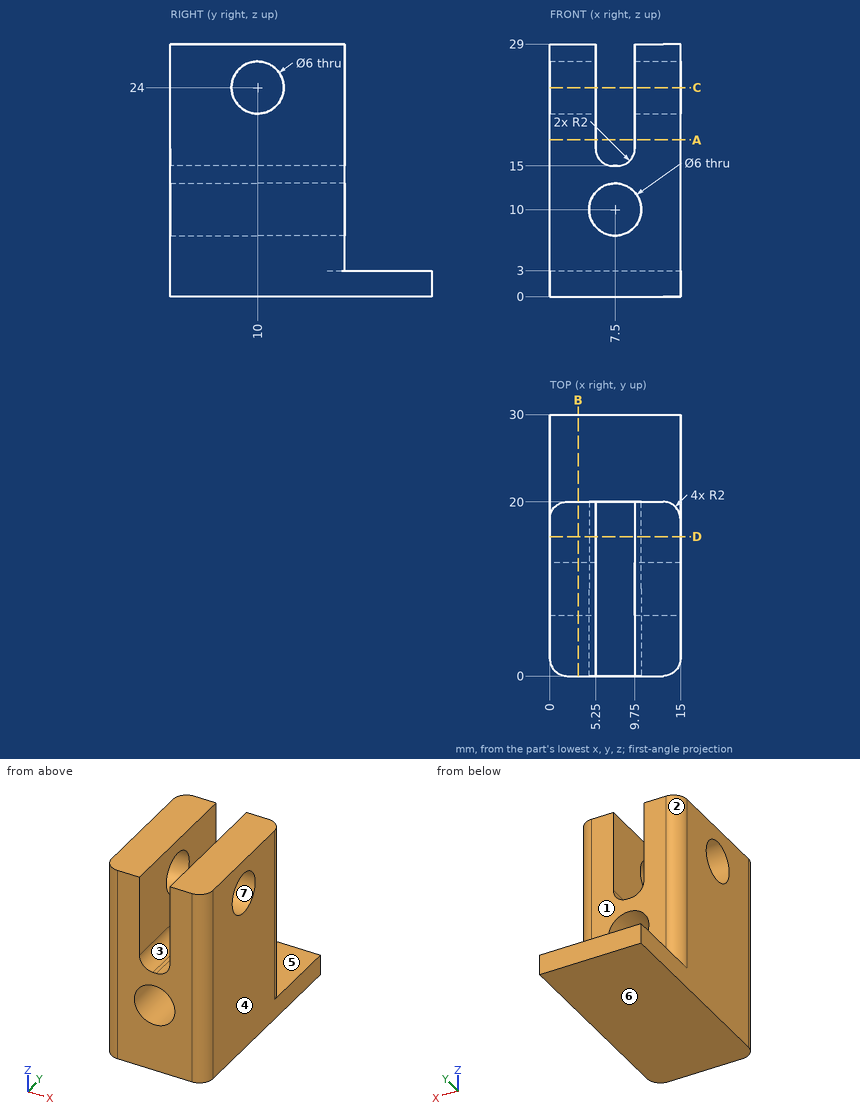
Print and shaded views of the part. All mm, measured from the part's lowest x, y and z. A direction names the side the tool comes from. Round coordinates to 2 decimals unless told otherwise and drop trailing zeros. Order: outer loops, then holes, each group sorted by start corner. A loop starts at its lowest first (then second) coordinate and runs counter-clockwise, first axis right, second up. Notation, with made-up numbers: (-38, 38.25) - (-14, 38.25) arc R35 ccw to (-14, 71.25) - close; hole circle Ø2 at (35.5, -25.75). An arc over 180 degrees is marked (long way). Use a Markdown table: item, result.
1) Saw through at C-C on z = 24. Write the cut outline in (x, y).
Recorded:
| item | result |
|---|---|
| outline | (0, 2) arc R2 ccw to (2, 0) - (5.25, 0) - (5.25, 7) - (0, 7) - close; (0, 13) - (5.25, 13) - (5.25, 20) - (2, 20) arc R2 ccw to (0, 18) - close; (9.75, 0) - (13, 0) arc R2 ccw to (15, 2) - (15, 7) - (9.75, 7) - close; (9.75, 13) - (15, 13) - (15, 18) arc R2 ccw to (13, 20) - (9.75, 20) - close |
2) Saw through at D-D on y = 16. Write the cut outline in (x, z), and give its area (3 significant figures).
Recorded:
| item | result |
|---|---|
| outline | (0, 0) - (15, 0) - (15, 29) - (9.75, 29) - (9.75, 17) arc R2 cw to (7.75, 15) - (7.25, 15) arc R2 cw to (5.25, 17) - (5.25, 29) - (0, 29) - close; hole circle Ø6 at (7.5, 10) |
| area | 345 mm² |
3) Tool access for the marked faces 1, 2 and 3: list every direction of +Z, -Z, +X, -X, +Y, -Y with a clear straight run to the whole face (end or side of a thin tool).
Recorded:
| item | result |
|---|---|
| face 1 | +Z, +X, -X, +Y |
| face 2 | +Z, -X, +Y |
| face 3 | +Z, +Y, -Y |
4) Saw through at B-B on x = 3.25. Write the cut outline in (y, z).
Recorded:
| item | result |
|---|---|
| outline | (0, 0) - (30, 0) - (30, 3) - (20, 3) - (20, 29) - (0, 29) - close; hole circle Ø6 at (10, 24) |
5) Saw through at A-A on z = 18. Write the cut outline in (x, y).
Recorded:
| item | result |
|---|---|
| outline | (0, 2) arc R2 ccw to (2, 0) - (5.25, 0) - (5.25, 20) - (2, 20) arc R2 ccw to (0, 18) - close; (9.75, 0) - (13, 0) arc R2 ccw to (15, 2) - (15, 18) arc R2 ccw to (13, 20) - (9.75, 20) - close |
6) Flat gauge pins, fed straight in: pin 1 Ø5.5 at (x, z) = (6, 12.5) entering from +Y; pin 2 Ø1 at (x, y) = (5.5, 22) entering from +Z. Where does each tip first touch, or does it go through?
Recorded:
| item | result |
|---|---|
| pin 1 | stops at y = 20 |
| pin 2 | stops at z = 3 |
7) Pull direction Z, two halves, no side cores. Call the marked faces 4, 5, 6 and 7: pulls with the +Z half, pulls with the -Z half, needs draft (parallel to the pull), parting line crosses it, or undercut.
Recorded:
| item | result |
|---|---|
| face 4 | needs draft |
| face 5 | pulls with the +Z half |
| face 6 | pulls with the -Z half |
| face 7 | undercut |
8) Wall check: L1, parallel to X at y = 2.25, z = 10; L2, parallel to Z at x = 2.55, y = 10; L3, parallel to X at y = 7, z = 23.25. Give the ranges that are in metal, low to high.
Recorded:
| item | result |
|---|---|
| L1 | x = 0 to 4.5, 10.5 to 15 |
| L2 | z = 0 to 21, 27 to 29 |
| L3 | x = 0 to 5.25, 9.75 to 15 |
